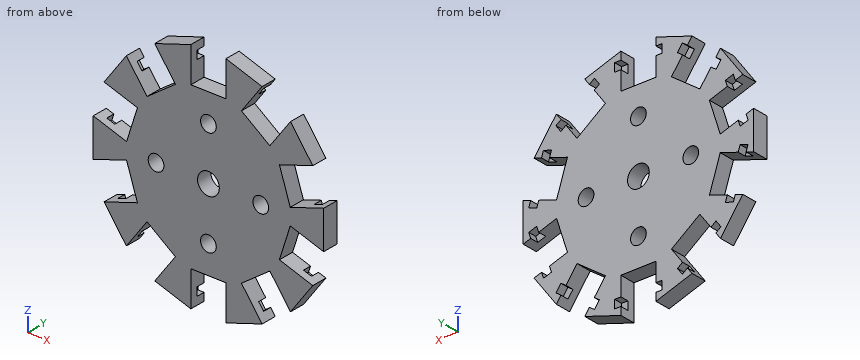
```python
from build123d import *

# Parameters (mm, degrees)
BOSS_EXTRUDE1_DEPTH = 3
CUT_EXTRUDE1_DEPTH  = 3
SKETCH7_R           = 1.5
CUT_EXTRUDE3_DEPTH  = 3
SKETCH4_W           = 9.1
SKETCH4_H           = 1.6
CUT_EXTRUDE2_DEPTH  = 1.6
SKETCH10_R          = 2.075
CUT_EXTRUDE6_DEPTH  = 3


with BuildPart() as part:
    # Sketch1 → Boss-Extrude1 (new body)
    with BuildSketch(Plane(origin=(0, 0, 0), x_dir=(1, 0, 0), z_dir=(0, 1, 0))):
        Polygon((0, 23.132168933), (-13.596747752, 18.714317784), (-22, 7.148233317), (-22, -7.148233317), (-13.596747752, -18.714317784), (0, -23.132168933), (13.596747752, -18.714317784), (22, -7.148233317), (22, 7.148233317), (13.596747752, 18.714317784), align=None)
    extrude(amount=BOSS_EXTRUDE1_DEPTH)

    # Sketch2 → Cut-Extrude1 (cut)
    with BuildSketch(Plane(origin=(0, 3, 0), x_dir=(1, 0, 0), z_dir=(0, 1, 0))):
        Polygon((0, 23.132168933), (-3.35, 22.043687951), (-3.35, 15.343687951), (3.35, 15.343687951), (3.35, 22.043687951), align=None)
        Polygon((11.729000424, 10.444223713), (15.667161615, 15.864637576), (13.596747752, 18.714317784), (10.246747752, 19.802798766), (6.308586562, 14.382384904), align=None)
        Polygon((15.627921341, 1.555421004), (22, 3.625834866), (22, 7.148233317), (19.929586138, 9.997913525), (13.557507479, 7.927499663), align=None)
        Polygon((13.557507479, -7.927499663), (19.929586138, -9.997913525), (22, -7.148233317), (22, -3.625834866), (15.627921341, -1.555421004), align=None)
        Polygon((6.308586562, -14.382384904), (10.246747752, -19.802798766), (13.596747752, -18.714317784), (15.667161615, -15.864637576), (11.729000424, -10.444223713), align=None)
        Polygon((-3.35, -15.343687951), (-3.35, -22.043687951), (0, -23.132168933), (3.35, -22.043687951), (3.35, -15.343687951), align=None)
        Polygon((-11.729000424, -10.444223713), (-15.667161615, -15.864637576), (-13.596747752, -18.714317784), (-10.246747752, -19.802798766), (-6.308586562, -14.382384904), align=None)
        Polygon((-15.627921341, -1.555421004), (-22, -3.625834866), (-22, -7.148233317), (-19.929586138, -9.997913525), (-13.557507479, -7.927499663), align=None)
        Polygon((-13.557507479, 7.927499663), (-19.929586138, 9.997913525), (-22, 7.148233317), (-22, 3.625834866), (-15.627921341, 1.555421004), align=None)
        Polygon((-6.308586562, 14.382384904), (-10.246747752, 19.802798766), (-13.596747752, 18.714317784), (-15.667161615, 15.864637576), (-11.729000424, 10.444223713), align=None)
    extrude(amount=-CUT_EXTRUDE1_DEPTH, mode=Mode.SUBTRACT)

    # Sketch7 → Cut-Extrude3 (cut)
    with BuildSketch(Plane(origin=(0, 3, 0), x_dir=(1, 0, 0), z_dir=(0, 1, 0))):
        with Locations(Location((0, 10, 0), (0, 0, 270))):
            Circle(SKETCH7_R)
        with Locations(Location((10, 0, 0), (0, 0, 270))):
            Circle(SKETCH7_R)
        with Locations(Location((0, -10, 0), (0, 0, 270))):
            Circle(SKETCH7_R)
        with Locations(Location((-10, 0, 0), (0, 0, 270))):
            Circle(SKETCH7_R)
    extrude(amount=-CUT_EXTRUDE3_DEPTH, mode=Mode.SUBTRACT)

    # Sketch4 → Cut-Extrude2 (cut)
    with BuildSketch(Plane(origin=(0, 3, 0), x_dir=(1, 0, 0), z_dir=(0, 1, 0))):
        with Locations((0, 19.743687951)):
            Rectangle(SKETCH4_W, SKETCH4_H)
        Polygon((7.453793077, 18.000188386), (8.394249481, 19.294615577), (15.75630413, 13.945769781), (14.815847726, 12.65134259), align=None)
        Polygon((16.610490544, 10.181228662), (18.13218097, 10.675655853), (20.944235619, 2.021041555), (19.422545193, 1.526614364), align=None)
        Polygon((19.422545193, -1.526614364), (20.944235619, -2.021041555), (18.13218097, -10.675655853), (16.610490544, -10.181228662), align=None)
        Polygon((14.815847726, -12.65134259), (15.75630413, -13.945769781), (8.394249481, -19.294615577), (7.453793077, -18.000188386), align=None)
        with Locations((0, -19.743687951)):
            Rectangle(SKETCH4_W, SKETCH4_H)
        Polygon((-7.453793077, -18.000188386), (-8.394249481, -19.294615577), (-15.75630413, -13.945769781), (-14.815847726, -12.65134259), align=None)
        Polygon((-16.610490544, -10.181228662), (-18.13218097, -10.675655853), (-20.944235619, -2.021041555), (-19.422545193, -1.526614364), align=None)
        Polygon((-19.422545193, 1.526614364), (-20.944235619, 2.021041555), (-18.13218097, 10.675655853), (-16.610490544, 10.181228662), align=None)
        Polygon((-14.815847726, 12.65134259), (-15.75630413, 13.945769781), (-8.394249481, 19.294615577), (-7.453793077, 18.000188386), align=None)
    extrude(amount=-CUT_EXTRUDE2_DEPTH, mode=Mode.SUBTRACT)

    # Sketch10 → Cut-Extrude6 (cut)
    with BuildSketch(Plane.XZ):
        with Locations(Location((0, 0, 0), (0, 0, 270))):
            Circle(SKETCH10_R)
    extrude(amount=-CUT_EXTRUDE6_DEPTH, mode=Mode.SUBTRACT)


solid = part.part
```
Geometry: final body of the model. Coordinates: model frame, mm. Round coordinates to 2 decimals unless told otherwise and drop trailing zeros. Order: outer loops, then holes, each group sorted by start corner. A loop starts at its lowest first (then second) coordinate and runs counter-clockwise, first axis right, second up. Notation, with made-up numbers: (23.5, 84) -> (53.5, 84) arc R7 cw to (53.5, 91) -> close; hole circle Ø1 at (24.5, -14.5). An arc over 180 degrees is marked (long way). Use one line per item in the form item = value. Start each with the question number.
1. Pin query (flat end, axial travel): pin 1 Ø0.6 at (x, y) = (4, 2.5) entering from +Z; pin 2 Ø1.3 at (y, z) = (2, -19.5) entering from +X; pin 3 Ø0.5 at (x, z) = (20, 2.5) entering from +Y. Return the tip coordinate at first contact, or that it passes through.
2. Cut plane A-A (x = 0). Return the cut outline in (y, z) (3 decimals).
3. Cut plane B-B (y = 0.7). Count the separate pieces of the cut face and the enclosed holes in it, then the cut area to 3 significant figures.
4. Line query: probe 1 along X at (y, z) = (2.2, 0) (3 decimals); probe 2 along Z at (x, y) = (19, 0.9); probe 3 along Z at (x, y) = (-19.5, 0.8). Output: solid intervals per line, ascending.
5. Cut plane C-C (z = -4.5). Return the cut outline in (x, y), then the cut area to 3 significant figures.
Solution:
q1.pin_1 = 21.93
q1.pin_2 = 10.25
q1.pin_3 = 1.4
q2.outline = (0, -15.344) -> (3, -15.344) -> (3, -11.5) -> (0, -11.5) -> close; (0, -8.5) -> (3, -8.5) -> (3, -2.075) -> (0, -2.075) -> close; (0, 2.075) -> (3, 2.075) -> (3, 8.5) -> (0, 8.5) -> close; (0, 11.5) -> (3, 11.5) -> (3, 15.344) -> (0, 15.344) -> close
q3.separate_pieces = 1
q3.enclosed_holes = 5
q3.area = 1,050 mm^2
q4.probe_1 = -22 to -11.5, -8.5 to -2.075, 2.075 to 8.5, 11.5 to 22
q4.probe_2 = -11.28 to -9.7, -2.65 to 2.65, 9.7 to 11.28
q4.probe_3 = -10.59 to -9.86, -2.81 to 2.81, 9.86 to 10.59
q5.outline = (-14.67, 0) -> (14.67, 0) -> (14.67, 3) -> (-14.67, 3) -> close
q5.area = 88.0 mm^2
